Build history of the part. All positions in model axes, mm. Face numbers are marked on the shaded views. A direction names the side the tool comes from. Coordinates: 2 decimals unless noted, no trailing zeros. Write each loop counter-clockwise with the first axis right and the second up, starting at its lowest first coordinate (ties: lowest second). Pieces come first, ordered by that corner, then holes. Notation, with made-up numbers: (10, 72.25) -> (49, 72.25) arc R10 ccw to (49, 76.25) -> close; hole circle Ø3 at (-20.75, 69.25). An arc over 180 degrees is marked (long way). Write each question's results on one line, items separated by ' | '. Start each with the question number.
Q1. Saw through at B-B on x = 12. Give the cut face in (y, z).
Q2. Drop flat-ended pins along their axis: pin 1 Ø4 at (x, z) = (2.5, -3.5) entering from +Y; pin 2 Ø1 at (x, y) = (2, 0) entering from +Z; pin 3 Ø2 at (x, y) = (7.5, -1.5) entering from +Z. Give the stop position or say it passes through.
Q3. Saw through at A-A on x = 7.75. Give the cut face in (y, z), and give its area (3 significant figures).
Q4. Tool access for the marked faces 1, 2 and 3: list every direction of +Z, -Z, +X, -X, +Y, -Y with a clear straight run to the whole face (end or side of a thin tool).
Q5. Drill centre lines: line 1 (X direction, y = -1.5, z = 2.25); line 2 (Y direction, x = 1.75, z = 0.5); line 3 (X direction, y = 0.75, z = 2.5). Where is each one in solid material? Low to high.
Q6. Two-plate mould, pull along Y, no slides. Class the marked faces 4, 5 and 6: released by +Y, released by -Y, zero draft, split by the parting line, or undercut.
Autodesk Inventor part; units mm, degrees
ref_plane "Work Plane2" through (3.3, 0, 0) normal (0, 0, 1) x (1, 0, 0)
ref_plane "YZ Plane" through (0, 0, 0) normal (1, 0, 0) x (0, 1, 0)
ref_plane "XZ Plane" through (0, 0, 0) normal (0, 1, 0) x (-1, 0, 0)
sketch "Sketch1" plane through (0, 0, 0) normal (0, 0, 1) x (1, 0, 0)
  line L0 (2.7625, 0) -> (13, 0)
  line L1 (13, 0) -> (13, 2.5)
  line L2 (13, 2.5) -> (4.7, 2.5)
  line L3 (4.7, 2.5) -> (4.2092, 2.0092)
  line L4 (4.2092, 2.0092) -> (3.6328, 2.0092)
  line L5 (0, 4.45) -> (0, 2.53)
  line L6 (0, 2.53) -> (1.9285, 1.5685)
  line L7 (1.9285, 1.5685) -> (2.7625, 0)
  line L8 (-2.6, 0) -> (15.6, 0)
  line L9 (0, -0.89) -> (0, 5.34)
  line L10 (0, 4.45) -> (0.66, 4.45)
  line L11 (0.66, 4.45) -> (2.7, 2.41)
  line L12 (2.7, 2.41) -> (3.4, 2.41)
  line L13 (3.4, 2.41) -> (3.6328, 2.0092)
  line L14 (3.4, 2.41) -> (4.61, 2.41) construction
  line L15 (4.7, 2.5) -> (2.61, 2.5) construction
  dimension "d0" = 8.3
  dimension "d1" = 5
  dimension "d2" = 4.0185
  dimension "d3" = 5.06
  dimension "d4" = 26.5
  dimension "d5" = 62
  dimension "d6" = 2.7625
  dimension "d11" = 8.9
  dimension "d12" = 4.82
  dimension "d13" = 45
  dimension "d14" = 59.85
  dimension "d15" = 2.7
  dimension "d17" = 0.7
  dimension "d19" = 13
  dimension "d27" = 45
revolve "Body" add sketch "Sketch1" angle 360 about axis through (2.7625, 0, 0) along (1, 0, 0) contours L7 L6 L5 L10 L11 L12 L13 L4 L3 L2 L1 L0
sketch "Sketch2" plane through (0, 0, 0) normal (-1, 0, 0) x (0, 0, 1)
  line L0 (0, 2.53) -> (0, 0) construction
  line L1 (0, 0) -> (2.53, 0) construction
  arc A0 (0.759, 0) -> (0, 0.759) centre (0, 0) ccw construction
  arc A1 (0.8855, 0) -> (0, 0.8855) centre (0, 0) ccw construction
  arc A2 (2.476, 0.52) -> (0.52, 2.476) centre (0, 0) ccw
  line L2 (0, 0) -> (1.789, 1.789) construction
  line L3 (0.52, 2.476) -> (0.4482, 0.7637)
  line L4 (2.476, 0.52) -> (0.7637, 0.4482)
  arc A3 (0.52, 2.476) -> (0, 2.53) centre (0, 0) ccw
  arc A4 (2.53, 0) -> (2.476, 0.52) centre (0, 0) ccw
  line L5 (0, -6.23) -> (0, 6.23)
  line L6 (-6.23, 0) -> (6.23, 0)
  arc A5 (0.52, -2.476) -> (2.476, -0.52) centre (0, 0) ccw
  line L7 (0.52, -2.476) -> (0.4482, -0.7637)
  line L8 (2.476, -0.52) -> (0.7637, -0.4482)
  arc A6 (0, -2.53) -> (0.52, -2.476) centre (0, 0) ccw
  arc A7 (2.476, -0.52) -> (2.53, 0) centre (0, 0) ccw
  arc A8 (-0.52, 2.476) -> (-2.476, 0.52) centre (0, 0) ccw
  line L9 (-0.52, 2.476) -> (-0.4482, 0.7637)
  line L10 (-2.476, 0.52) -> (-0.7637, 0.4482)
  arc A9 (0, 2.53) -> (-0.52, 2.476) centre (0, 0) ccw
  arc A10 (-2.476, 0.52) -> (-2.53, 0) centre (0, 0) ccw
  arc A11 (-0.52, -2.476) -> (0, -2.53) centre (0, 0) ccw
  arc A12 (-2.476, -0.52) -> (-0.52, -2.476) centre (0, 0) ccw
  arc A13 (-2.53, 0) -> (-2.476, -0.52) centre (0, 0) ccw
  line L11 (-2.476, -0.52) -> (-0.7637, -0.4482)
  line L12 (-0.52, -2.476) -> (-0.4482, -0.7637)
  arc A14 (0.4482, 0.7637) -> (0.7637, 0.4482) centre (0.751, 0.751) ccw
  arc A15 (0.7637, -0.4482) -> (0.4482, -0.7637) centre (0.751, -0.751) ccw
  arc A16 (-0.7637, 0.4482) -> (-0.4482, 0.7637) centre (-0.751, 0.751) ccw
  arc A17 (-0.4482, -0.7637) -> (-0.7637, -0.4482) centre (-0.751, -0.751) ccw
  point P0 (1.789, -1.789)
  point P1 (-1.789, 1.789)
  point P2 (-1.789, -1.789)
  dimension "d20" = 1.518
  dimension "d21" = 1.771
  dimension "d22" = 5.06
  dimension "d23" = 45
  dimension "d24" = 0.52
extrude "Slot" add sketch "Sketch2" against normal up to next draft 5 contours L4 A14 L3 A2 | A5 L7 A15 L8 | L9 A16 L10 A8 | A12 L11 A17 L12
fillet "Fillet1" radius 0.208 4 edges at (0, 2.53, 0) (0, 0, -2.53) (0, -2.53, 0) (0, 0, 2.53)
thread "Thread"
chamfer "Chamfer1" distance 0.53 distance2 2.8 1 edges at (13, -2.5, 0) measured on face at (13, -0.5525, -0.0341)
ref_plane "Work Plane2" through (3.3, 0, 0) normal (0, 0, 1) x (1, 0, 0)
equation "\"d20\" = 0.3 * SDM"
equation "\"d21\" = 0.35 * SDM"
equation "\"d22\" = SDM"
equation "\"d24\" = 0.5 * SBR"
equation "\"d0\" = GEL"
equation "\"d1\" = NND"
equation "\"d2\" = GD1"
equation "\"d3\" = SDM"
equation "\"d6\" = 0.85 * INTI"
equation "\"d11\" = KOD"
equation "\"d12\" = SD2"
equation "\"d13\" = 0.5 * SEWI"
equation "\"d14\" = 1.33 * ANGL"
equation "\"d15\" = KOH"
equation "\"d17\" = SD"
equation "\"d19\" = NLG"
equation "\"d27\" = ANGL"
equation "\"d26\" = 0.2 * SBR"
equation "\"d8\" = GEL"
equation "\"d28\" = -0.5 * GD2 + 0.5 * NND"
equation "\"d29\" = SPTZ"
equation "\"NLG\" = 13"
equation "\"GEL\" = 8.3"
equation "\"GD2\" = 3.94"
equation "\"KOD\" = 8.9"
equation "\"KOH\" = 2.7"
equation "\"SBR\" = 1.04"
equation "\"INTI\" = 3.25"
equation "\"SDM\" = 5.06"
equation "\"NND\" = 5"
equation "\"GD1\" = THREADDIA - 1.2269 * PTC"
equation "\"SEWI\" = 90deg"
equation "\"d7\" = SDM"
equation "\"ANGL\" = 45deg"
equation "\"SD\" = 0.7"
equation "\"SD2\" = 4.82"
equation "\"SPTZ\" = 2.8"
equation "\"TOA\" = 30deg"
equation "\"THREADDIA\" = 5"
equation "\"PTC\" = 0.8"
equation "\"GUL\" = 0.61345 * PTC"
equation "\"GAL\" = 0.61345 * PTC"
properties part number "ANSI B18.6.5M - M5x0.8 x 13 - D - I" material "Steel, Mild"
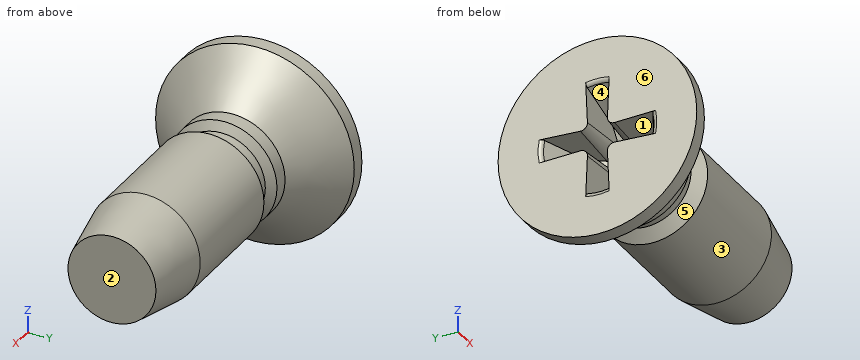
Returned:
1) outline: circle Ø4.32 at (0, 0)
2) pin 1: stops at y = 3.55 | pin 2: stops at z = 3.61 | pin 3: stops at z = 2.45
3) outline: circle Ø5 at (0, 0) | area: 19.6 mm2
4) face 1: -X | face 2: +Z, -Z, +X, +Y, -Y | face 3: +X
5) line 1: x = 0 to 2.41 | line 2: y = -3.32 to -0.37, 0.37 to 3.32 | line 3: x = 0 to 2.5
6) face 4: undercut | face 5: split by the parting line | face 6: zero draft
